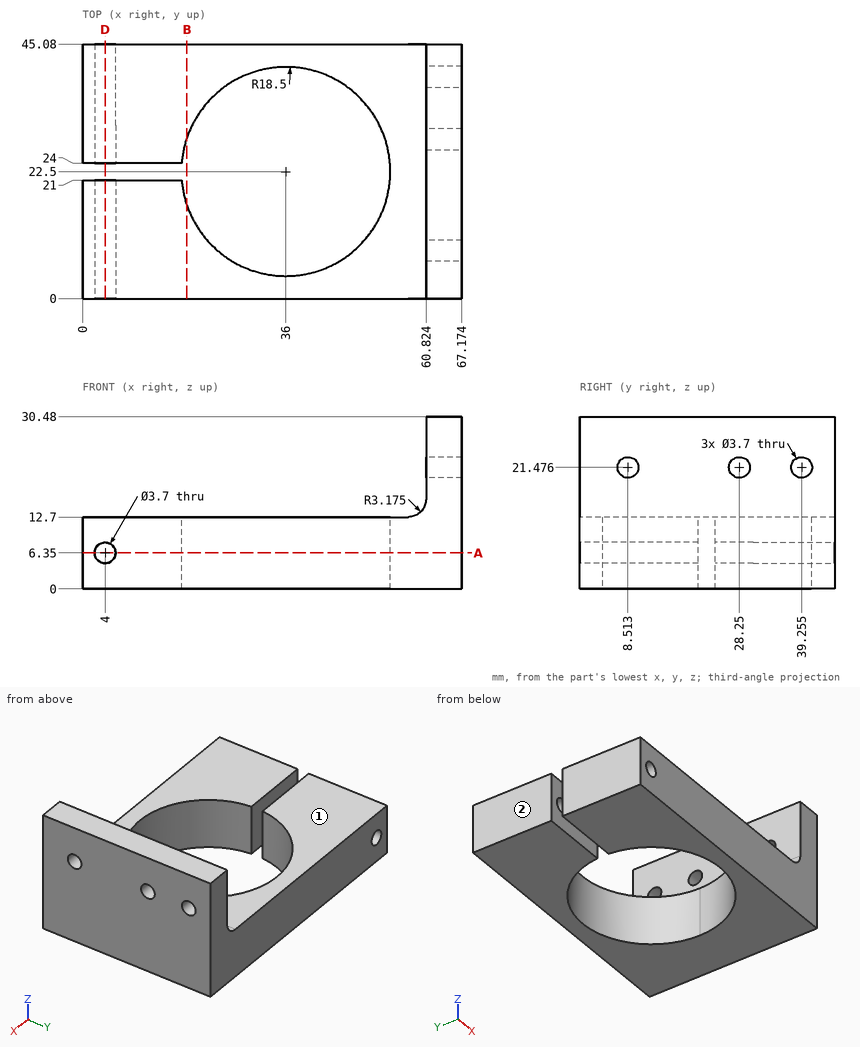
Geometry check sheet. Reference: drawing and pictorial views, mm from the part's lowest x, y, z. A direction names the side the tool comes from. Give positions to 0.01 mm unless a question says otherwise; leave off trailing zeros. Order: outer loops, then holes, each group sorted by start corner. A loop starts at its lowest first (then second) coordinate and runs counter-clockwise, first axis right, second up. Notation, with made-up numbers: M 71.5,35 L 98.5,35 A33 cw 98.5,66 Z; hole C 28,-1.75 d2. An arc over 180 degrees is marked long. Answer as a JSON object with one key per item and string values. Group by question number.
1) Cross-section at A-A (z = 6.35). Give the number of separate pieces and of enclosed holes in the cut face.
2) Cross-section at D-D (x = 4). Enter the section's corners in (y, z), then the cut area to 3 significant figures.
3) Access from +Z, -Z, +X, -X, +Y, -Y to the whole of each face (thin tool, end or side, straight path). Record for the marked faces 1 and 2.
4) Depth check by flat-ended pin: pin 1 Ø8 at (y, z) = (10, 21.5) entering from -X; pin 2 Ø8 at (x, y) = (54, 31) entering from -Z; pin 3 Ø3 at (x, z) = (4, 6.35) entering from +Y; pin 4 Ø1.5 at (x, y) = (59.5, 38) entering from +Z (1 decimal). Enter the tip coordinate at first touch or a pass-through.
5) Scan lines: line 1 along X through (y, z) = (6.5, 7) (1 decimal); line 2 along Y through (x, z) = (11.5, 7); line 3 along X through (y, z) = (8, 5) (1 decimal). Record each from-to range of solid material in increasing order. Write a range as [from, to].
6) Cross-section at B-B (x = 18.5). Enter the section's corners in (y, z).
Result sheet:
{
 "1": {"separate pieces": "3", "enclosed holes": "0"},
 "2": {"outline": "M 0,0 L 21,0 L 21,4.5 L 0,4.5 Z; M 0,8.2 L 21,8.2 L 21,12.7 L 0,12.7 Z; M 24,0 L 45.08,0 L 45.08,4.5 L 24,4.5 Z; M 24,8.2 L 45.08,8.2 L 45.08,12.7 L 24,12.7 Z", "area": "379 mm2"},
 "3": {"face 1": "+Z, -X, +Y, -Y", "face 2": "+Z, -Z, -X, +Y, -Y"},
 "4": {"pin 1": "stops at x = 60.82", "pin 2": "stops at z = 0", "pin 3": "passes through", "pin 4": "stops at z = 14.1"},
 "5": {"line 1": "x = [0, 2.3], [5.7, 26.7], [45.3, 67.2]", "line 2": "y = [0, 21], [24, 45.08]", "line 3": "x = [0, 2.7], [5.3, 24.5], [47.5, 67.2]"},
 "6": {"outline": "M 0,0 L 16.5,0 L 16.5,12.7 L 0,12.7 Z; M 28.5,0 L 45.08,0 L 45.08,12.7 L 28.5,12.7 Z"}
}
